```python
from build123d import *

# Parameters (mm, degrees)
EXTRUDE_1_DEPTH      = 1
EXTRUDE_1_DEPTH_BACK = 1
SKETCH_1_W           = 27.72
SKETCH_1_H           = 27.72
SKETCH_1_5_W         = 31.52
SKETCH_1_5_H         = 33.72
SKETCH_1_5_W_2       = 27.72
SKETCH_1_5_H_2       = 27.72
EXTRUDE_3_DEPTH      = 1


with BuildPart() as part:
    # 草图1 → 凸台-拉伸1 (new, two sides: drawn at the far end of the back side and taken through both)
    with BuildSketch(Plane.XY.offset(-EXTRUDE_1_DEPTH_BACK)):
        Rectangle(SKETCH_1_W, SKETCH_1_H)
    extrude(amount=EXTRUDE_1_DEPTH + EXTRUDE_1_DEPTH_BACK)

    # 草图1<5> → 凸台-拉伸3 (add)
    with BuildSketch(Plane.XY):
        with Locations((0, -1.5)):
            Rectangle(SKETCH_1_5_W, SKETCH_1_5_H)
        Rectangle(SKETCH_1_5_W_2, SKETCH_1_5_H_2, mode=Mode.SUBTRACT)
    extrude(amount=-EXTRUDE_3_DEPTH)


solid = part.part
```
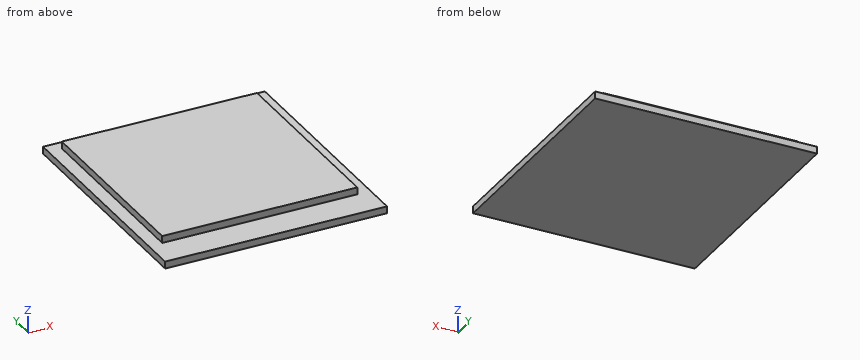
CAD build for the part. Positions are in the model's coordinates, mm. Coordinates: 2 decimals unless noted, no trailing zeros. Order: outer loops, then holes, each group sorted by start corner. A loop starts at its lowest first (then second) coordinate and runs counter-clockwise, first axis right, second up. Notation, with made-up numbers: (36.5, 65) - (57.5, 65) arc R30 ccw to (57.5, 99) - close; hole circle Ø3 at (9, -15). An arc over 180 degrees is marked (long way). Use a Markdown table: item, result. Add a question column.
(1) Flat gauge pin, fed straight in: pin 1 (0.5 mm diameter, centred on x = -5, z = 0.5, fed in from -Y). Where does the tip first touch, or does it go through?
(2) Saw through at B-B (y = 9). Give the cut face in (x, z), then the cut area to 3 significant figures.
(3) Saw through at C-C (z = 0.45). Give the cut face in (x, y), then the cut area to 3 significant figures.
(4) Saw through at A-A (x = -10). Give the cut face in (y, z), then the cut area to 3 significant figures.
(5) Drill centre lines: line 1 along Y through (x, z) = (11.5, 0.85); line 2 along Z through (x, y) = (-4, -15). Where is each one in solid material? Low to high. Write a range as [from, to].
Solved:
| question | item | result |
|---|---|---|
| 1 | pin 1 | stops at y = -13.86 |
| 2 | outline | (-15.76, -1) - (15.76, -1) - (15.76, 0) - (13.86, 0) - (13.86, 1) - (-13.86, 1) - (-13.86, 0) - (-15.76, 0) - close |
| 2 | area | 59.2 mm² |
| 3 | outline | (-13.86, -13.86) - (13.86, -13.86) - (13.86, 13.86) - (-13.86, 13.86) - close |
| 3 | area | 768 mm² |
| 4 | outline | (-18.36, -1) - (15.36, -1) - (15.36, 0) - (13.86, 0) - (13.86, 1) - (-13.86, 1) - (-13.86, 0) - (-18.36, 0) - close |
| 4 | area | 61.4 mm² |
| 5 | line 1 | y = [-13.86, 13.86] |
| 5 | line 2 | z = [-1, 0] |
